Build history of the part. All positions in model axes, mm. A direction names the side the tool comes from. Coordinates: 2 decimals unless noted, no trailing zeros. Order: outer loops, then holes, each group sorted by start corner. A loop starts at its lowest first (then second) coordinate and runs counter-clockwise, first axis right, second up. Notation, with made-up numbers: (77.25, -15) - (110.25, -15) arc R30 ccw to (110.25, 15) - close; hole circle Ø10 at (47, 65). An arc over 180 degrees is marked (long way). Return JSON: item names as keys, results as strings.
from build123d import *

# Parameters (mm, degrees)
SKETCH1_W           = 20
SKETCH1_H           = 13
BOSS_EXTRUDE1_DEPTH = 16
SKETCH2_R           = 1.95
BOSS_EXTRUDE2_DEPTH = 9.652509653
SKETCH3_R           = 3
BOSS_EXTRUDE3_DEPTH = 12.895752896
SKETCH4_W           = 1
SKETCH4_H           = 3
CUT_EXTRUDE1_DEPTH  = 1


with BuildPart() as part:
    # Sketch1 → Boss-Extrude1 (new body)
    with BuildSketch(Plane(origin=(0, 0, 0), x_dir=(1, 0, 0), z_dir=(0, 1, 0))):
        Rectangle(SKETCH1_W, SKETCH1_H)
    extrude(amount=BOSS_EXTRUDE1_DEPTH)

    # Sketch2 → Boss-Extrude2 (add)
    with BuildSketch(Plane.ZY.offset(10)):
        with Locations((0, 8)):
            Circle(SKETCH2_R)
    extrude(amount=BOSS_EXTRUDE2_DEPTH)

    # Sketch3 → Boss-Extrude3 (add)
    with BuildSketch(Plane(origin=(10, 0, 0), x_dir=(0, 0, -1), z_dir=(1, 0, 0))):
        with Locations((0, 8)):
            Circle(SKETCH3_R)
    extrude(amount=BOSS_EXTRUDE3_DEPTH)

    # Sketch4 → Cut-Extrude1 (cut)
    with BuildSketch(Plane.XY.offset(6.5)):
        with Locations((-9.5, 8)):
            Rectangle(SKETCH4_W, SKETCH4_H)
    extrude(amount=-CUT_EXTRUDE1_DEPTH, mode=Mode.SUBTRACT)


solid = part.part
1. Cut at C-C on x = -11. Give the cut face in (y, z).
Check values:
{"outline": "circle Ø3.9 at (8, 0)"}
2. Cut at D-D on y = 11.75. Give the cut face in (x, z).
Check values:
{"outline": "(-10, -6.5) - (10, -6.5) - (10, 6.5) - (-10, 6.5) - close"}
3. Cut at B-B on y = 8. Give the cut face in (x, z).
Check values:
{"outline": "(-19.65, -1.95) - (-10, -1.95) - (-10, -6.5) - (10, -6.5) - (10, -3) - (22.9, -3) - (22.9, 3) - (10, 3) - (10, 6.5) - (-9, 6.5) - (-9, 5.5) - (-10, 5.5) - (-10, 1.95) - (-19.65, 1.95) - close"}
4. Drop flat-ended pins along their axis: pin 1 (5 mm diameter, centred on x = -13.5, y = 11, fed in from +Z); pin 2 (0.8 mm diameter, centred on y = 7.5, z = 6, fed in from -X); pin 3 (4 mm diameter, centred on y = 4.5, z = 4, fed in from +X). Give the stop position or say it passes through.
Check values:
{"pin 1": "z = 1.88", "pin 2": "x = -9", "pin 3": "x = 10"}
5. Cut at A-A on z = 0. Give the cut face in (x, y).
Check values:
{"outline": "(-19.65, 6.05) - (-10, 6.05) - (-10, 0) - (10, 0) - (10, 5) - (22.9, 5) - (22.9, 11) - (10, 11) - (10, 16) - (-10, 16) - (-10, 9.95) - (-19.65, 9.95) - close"}
6. Probe L1, parallel to X at y = 1.5, z = -3.25; L2, parallel to X at y = 10.75, z = 0; L3, parallel to Z at x = -9.5, y = 8.75. List the from-to ranges inside material, lowest first.
Check values:
{"L1": "-10 to 10", "L2": "-10 to 22.9", "L3": "-6.5 to 5.5"}
7. Tool access for faces 1 (the flat face through (0, 0, 0)), 2 (the flat face through (22.896, 8, 0)), 3 (the flat face through (-9.5, 6.5, 6)), 4 (the cylindrical face through (16.36, 10.53, -1.61)), 5 (the cylindrical face through (-14.759, 9.933, -0.254)): list every direction of +Z, -Z, +X, -X, +Y, -Y with a clear straight run to the whole face (end or side of a thin tool).
Check values:
{"face 1": "+Z, -Z, +X, -X, -Y", "face 2": "+Z, -Z, +X, +Y, -Y", "face 3": "+Z, -X", "face 4": "+X", "face 5": "-X"}
